Model file for the job. Use its own axes, mm. A direction names the side the tool comes from. Give positions to 0.01 mm unless a question says otherwise; leave off trailing zeros. Write each loop counter-clockwise with the first axis right and the second up, starting at its lowest first coordinate (ties: lowest second). Pieces come first, ordered by that corner, then holes. Notation, with made-up numbers: (-22, 8) - (1, 8) arc R22 cw to (1, 36) - close; hole circle Ø3 at (51.5, 13.5). An arc over 180 degrees is marked (long way). One line per item, written item: value. Start each with the question number.
(1) Probe L1, parallel to Z at x = -0.25, y = -0.35; L2, parallel to X at y = -0.35, z = 0.5; L3, parallel to Y at x = 3.25, z = 2.25. List the from-to ranges inside material, lowest first.
(2) 3-axis set-ups, long thin cutter, end or side, ignore diameter. For faces 4 (the face through (-8.26, 0.986, 5.634)), 5 (the face through (9.3, 1, 0)), 6 (the face through (-10, 1, -3.5)), 7 (the face through (0, -1, 4.25)), 8 (the face through (9, -1, 0)): which of +Z, -Z, +X, -X, +Y, -Y reach the whole face in a straight line?
(3) Cut at C-C, the plane z = -0.5. List the corners of the cut face in (x, y).
(4) Cut at B-B, the plane x = -2.5. List the corners of the cut face in (y, z), and give its area (3 significant figures).
(5) Drop flat-ended pins along their axis: P1, Ø7, axis at x = -2, z = 0.5, coming from the -Y side; P2, Ø1, axis at x = 4, y = 1, coming from the -Z side; P3, Ø1.1, axis at x = 10, y = 1, coming from the +Z side; P4, Ø1.1, axis at x = 9.5, y = 1, coming from the -Z side. Give the stop position or say it passes through.
(6) Mould opens along Y. For faces 1 (the face through (10, 1, -3.5)), 2 (the face through (-7.8, -1.48, -3.82)), 3 (the face through (10, 0, 0)) say: pulls with the +Y half, pulls with the -Y half, needs draft (parallel to the pull), parting line crosses it, or undercut.
(7) Cut at D-D, the plane z = -5.5. List the corners of the cut face in (x, y).
(8) Cut at A-A, the plane y = -1.35. List the corners of the cut face in (x, z), and give its area (4 significant figures).
from build123d import *

# Parameters (mm, degrees)
BOSS_EXTRUDE1_DEPTH      = 2
BOSS_EXTRUDE1_DEPTH_BACK = 3
BOSS_EXTRUDE2_DEPTH      = 2
BOSS_EXTRUDE3_DEPTH      = 2
SKETCH3_W                = 7
SKETCH3_H                = 1
CUT_EXTRUDE2_DEPTH       = 1.2
SKETCH4_W                = 7
SKETCH4_H                = 1
CUT_EXTRUDE3_DEPTH       = 1.2


with BuildPart() as part:
    # Sketch2 → Boss-Extrude1 (new body, two sides)
    with BuildSketch(Plane(origin=(0, 0, 0), x_dir=(1, 0, 0), z_dir=(0, 1, 0))) as boss_extrude1_sk:
        with BuildLine():
            Line((-7.5, 5), (7.5, 5))
            ThreePointArc((7.5, 5), (8.560660172, 4.560660172), (9, 3.5))
            Line((9, 3.5), (9, -3.5))
            ThreePointArc((9, -3.5), (8.560660172, -4.560660172), (7.5, -5))
            Line((7.5, -5), (-7.5, -5))
            ThreePointArc((-7.5, -5), (-8.560660172, -4.560660172), (-9, -3.5))
            Line((-9, -3.5), (-9, 3.5))
            ThreePointArc((-9, 3.5), (-8.560660172, 4.560660172), (-7.5, 5))
        make_face()
        with BuildLine():
            Line((-8.25, 2.75), (-8.25, -2.75))
            ThreePointArc((-8.25, -2.75), (-7.810660172, -3.810660172), (-6.75, -4.25))
            Line((-6.75, -4.25), (6.75, -4.25))
            ThreePointArc((6.75, -4.25), (7.810660172, -3.810660172), (8.25, -2.75))
            Line((8.25, -2.75), (8.25, 2.75))
            ThreePointArc((8.25, 2.75), (7.810660172, 3.810660172), (6.75, 4.25))
            Line((6.75, 4.25), (-6.75, 4.25))
            ThreePointArc((-6.75, 4.25), (-7.810660172, 3.810660172), (-8.25, 2.75))
        make_face(mode=Mode.SUBTRACT)
    extrude(amount=BOSS_EXTRUDE1_DEPTH)
    extrude(boss_extrude1_sk.sketch, amount=-BOSS_EXTRUDE1_DEPTH_BACK)

    # Sketch2_3 → Boss-Extrude2 (add)
    with BuildSketch(Plane(origin=(0, 0, 0), x_dir=(1, 0, 0), z_dir=(0, 1, 0))):
        with BuildLine():
            ThreePointArc((-8.25, 2.75), (-7.810660172, 3.810660172), (-6.75, 4.25))
            Line((-6.75, 4.25), (6.75, 4.25))
            ThreePointArc((6.75, 4.25), (7.810660172, 3.810660172), (8.25, 2.75))
            Line((8.25, 2.75), (8.25, -2.75))
            ThreePointArc((8.25, -2.75), (7.810660172, -3.810660172), (6.75, -4.25))
            Line((6.75, -4.25), (-6.75, -4.25))
            ThreePointArc((-6.75, -4.25), (-7.810660172, -3.810660172), (-8.25, -2.75))
            Line((-8.25, -2.75), (-8.25, 2.75))
        make_face()
    extrude(amount=BOSS_EXTRUDE2_DEPTH)

    # Sketch2_4 → Boss-Extrude3 (add)
    with BuildSketch(Plane(origin=(0, 0, 0), x_dir=(1, 0, 0), z_dir=(0, 1, 0))):
        with BuildLine():
            Line((-7.5, 5), (-9, 6.25))
            ThreePointArc((-9, 6.25), (-10.060660172, 5.810660172), (-10.5, 4.75))
            Line((-10.5, 4.75), (-10.5, -4.75))
            ThreePointArc((-10.5, -4.75), (-10.060660172, -5.810660172), (-9, -6.25))
            Line((-9, -6.25), (-7.5, -5))
            ThreePointArc((-7.5, -5), (-8.560660172, -4.560660172), (-9, -3.5))
            Line((-9, -3.5), (-9, 3.5))
            ThreePointArc((-9, 3.5), (-8.560660172, 4.560660172), (-7.5, 5))
        make_face()
        with BuildLine():
            Line((9, 6.25), (7.5, 5))
            ThreePointArc((7.5, 5), (8.560660172, 4.560660172), (9, 3.5))
            Line((9, 3.5), (9, -3.5))
            ThreePointArc((9, -3.5), (8.560660172, -4.560660172), (7.5, -5))
            Line((7.5, -5), (9, -6.25))
            ThreePointArc((9, -6.25), (10.060660172, -5.810660172), (10.5, -4.75))
            Line((10.5, -4.75), (10.5, 4.75))
            ThreePointArc((10.5, 4.75), (10.060660172, 5.810660172), (9, 6.25))
        make_face()
    extrude(amount=BOSS_EXTRUDE3_DEPTH)

    # Sketch3 → Cut-Extrude2 (cut)
    with BuildSketch(Plane.ZY.offset(10.5)):
        with Locations((0, 1)):
            Rectangle(SKETCH3_W, SKETCH3_H)
    extrude(amount=-CUT_EXTRUDE2_DEPTH, mode=Mode.SUBTRACT)

    # Sketch4 → Cut-Extrude3 (cut)
    with BuildSketch(Plane(origin=(10.5, 0, 0), x_dir=(0, 0, -1), z_dir=(1, 0, 0))):
        with Locations((0, 1)):
            Rectangle(SKETCH4_W, SKETCH4_H)
    extrude(amount=-CUT_EXTRUDE3_DEPTH, mode=Mode.SUBTRACT)


solid = part.part
Answers follow:
1. L1: z = -5 to -4.25, 4.25 to 5
1. L2: x = -9 to -8.25, 8.25 to 9
1. L3: y = 0 to 2
2. face 4: +Z, +Y, -Y
2. face 5: +X
2. face 6: -X
2. face 7: -Y
2. face 8: +Z, -Z, +X, -Y
3. outline: (-10.5, 0) - (-9, 0) - (-9, -3) - (-8.25, -3) - (-8.25, 0) - (8.25, 0) - (8.25, -3) - (9, -3) - (9, 0) - (10.5, 0) - (10.5, 0.5) - (9.3, 0.5) - (9.3, 1.5) - (10.5, 1.5) - (10.5, 2) - (-10.5, 2) - (-10.5, 1.5) - (-9.3, 1.5) - (-9.3, 0.5) - (-10.5, 0.5) - close
4. outline: (-3, -5) - (2, -5) - (2, 5) - (-3, 5) - (-3, 4.25) - (0, 4.25) - (0, -4.25) - (-3, -4.25) - close
4. area: 24.5 mm²
5. P1: stops at y = 0
5. P2: stops at z = -5
5. P3: stops at z = 6.18
5. P4: stops at z = -6.25
6. face 1: undercut
6. face 2: needs draft
6. face 3: pulls with the -Y half
7. outline: (-10.3, 0) - (-8.1, 0) - (-8.1, 2) - (-10.3, 2) - close; (8.1, 0) - (10.3, 0) - (10.3, 2) - (8.1, 2) - close
8. outline: (-9, -3.5) arc R1.5 ccw to (-7.5, -5) - (7.5, -5) arc R1.5 ccw to (9, -3.5) - (9, 3.5) arc R1.5 ccw to (7.5, 5) - (-7.5, 5) arc R1.5 ccw to (-9, 3.5) - close; hole (-8.25, -2.75) arc R1.5 ccw to (-6.75, -4.25) - (6.75, -4.25) arc R1.5 ccw to (8.25, -2.75) - (8.25, 2.75) arc R1.5 ccw to (6.75, 4.25) - (-6.75, 4.25) arc R1.5 ccw to (-8.25, 2.75) - close
8. area: 39.75 mm²
